For this review, take the finished solid that the model builds, in its own axes (mm). A direction names the side the tool comes from. Coordinates: 2 decimals unless noted, no trailing zeros. Loops run counter-clockwise (first coordinate to the right, second up) from the corner with the lowest first, then second, coordinate; pieces in that order, holes last. Notation, with made-up numbers: M 63,44 L 117,44 A25 ccw 117,69 Z; hole C 33.25,-21.75 d9. An arc over 180 degrees is marked long. Answer as a JSON object with one key per item and string values. Group by question number.
Item 1: Add section D-D (x = 28.5). State the section outline as (y, z) points.
Item 2: Wall thickness on L1, parallel to Z at x = -4, y = 30.5; L2, parallel to Z at x = 0, y = 6.8; L3, parallel to X at y = 8, z = 217: over which ranges is each line inside the solid? List them lowest first. Write a range as from..to.
Item 3: Mouldability with a two-part tool opening along Z and no side actions: class faces 5 (the face through (0, 0, 230)), 6 (the face through (0, 50, 2)), 7 (the face through (0, 30, 5)) as +Z half, -Z half, draft (parallel to the pull), parting line (faces both ways), or undercut.
Item 4: Insertion check: pin 1 (1.5 mm diameter, centred on y = 38.5, z = 26, fed in from +X); pin 2 (2.5 mm diameter, centred on y = 13.5, z = 72, fed in from -X); pin 3 (16.5 mm diameter, centred on x = 2, z = 158, fed in from +Y); pin 4 (5.5 mm diameter, centred on x = -36, z = 31.5, fed in from -Y). Each pin has a flat end and moves straight along its axis. Give the tip position at first contact, or say it passes through.
Item 5: Tool access review of faces 1 (the face through (0, 10, 151)), 2 (the face through (32.5, 16, 2)), 3 (the face through (32.5, 44, 2)), 4 (the face through (32.5, 30, 38)): name each direction out of +Z, -Z, +X, -X, +Y, -Y from which nothing blocks a thin tool from reaching the whole face with its end or side.
Item 6: Add section A-A (y = 0). State the section outline as (x, z) points, then the cut area to 3 significant figures.
Item 7: Add section B-B (z = 50). State the section outline as (x, y) points, then the cut area to 3 significant figures.
Item 8: Add section C-C (y = 34.5). State the section outline as (x, z) points.
from build123d import *

# Parameters (mm, degrees)
SKETCH1_W            = 15
SKETCH1_H            = 20
BOSS_EXTRUDE1_DEPTH  = 230
SKETCH2_W            = 65
SKETCH2_H            = 40
BOSS_EXTRUDE6_DEPTH  = 5
SKETCH7_W            = 75
SKETCH7_H            = 15
BOSS_EXTRUDE7_DEPTH  = 5
SKETCH8_W            = 75
SKETCH8_H            = 15
BOSS_EXTRUDE8_DEPTH  = 5
SKETCH9_W            = 65
SKETCH9_H            = 40
BOSS_EXTRUDE11_DEPTH = 5
CUT_EXTRUDE1_DEPTH   = 240.635139326
SKETCH13_R           = 1.984375
CUT_EXTRUDE2_DEPTH   = 10


with BuildPart() as part:
    # Sketch1 → Boss-Extrude1 (new body)
    with BuildSketch(Plane.XY):
        Rectangle(SKETCH1_W, SKETCH1_H)
    extrude(amount=BOSS_EXTRUDE1_DEPTH)

    # Sketch2 → Boss-Extrude6 (add)
    with BuildSketch(Plane(origin=(0, 0, 0), x_dir=(-1, 0, 0), z_dir=(0, 0, -1))):
        with Locations((0, 30)):
            Rectangle(SKETCH2_W, SKETCH2_H)
    extrude(amount=-BOSS_EXTRUDE6_DEPTH)

    # Sketch7 → Boss-Extrude7 (add)
    with BuildSketch(Plane(origin=(32.5, 0, 0), x_dir=(0, 0, -1), z_dir=(1, 0, 0))):
        with Locations((-37.5, 30)):
            Rectangle(SKETCH7_W, SKETCH7_H)
    extrude(amount=BOSS_EXTRUDE7_DEPTH)

    # Sketch8 → Boss-Extrude8 (add)
    with BuildSketch(Plane.ZY.offset(32.5)):
        with Locations((37.5, 30)):
            Rectangle(SKETCH8_W, SKETCH8_H)
    extrude(amount=BOSS_EXTRUDE8_DEPTH)

    # Sketch9 → Boss-Extrude11 (add)
    with BuildSketch(Plane.XY.offset(75)):
        with Locations((0, 30)):
            Rectangle(SKETCH9_W, SKETCH9_H)
    extrude(amount=-BOSS_EXTRUDE11_DEPTH)

    # Sketch10 → Cut-Extrude1 (cut, through all)
    with BuildSketch(Plane.ZY.offset(7.5)):
        with BuildLine():
            Line((209.843145751, 2), (211.343145751, 2))
            ThreePointArc((211.343145751, 2), (223, 0), (211.343145751, -2))
            Line((211.343145751, -2), (209.843145751, -2))
            Line((209.843145751, -2), (209.843145751, 2))
        make_face()
    extrude(amount=-CUT_EXTRUDE1_DEPTH, mode=Mode.SUBTRACT)

    # Sketch13 → Cut-Extrude2 (cut)
    with BuildSketch(Plane(origin=(0, 10, 0), x_dir=(1, 0, 0), z_dir=(0, 1, 0))):
        with Locations(Location((0, -217, 0), (0, 0, 270))):
            Circle(SKETCH13_R)
    extrude(amount=-CUT_EXTRUDE2_DEPTH, mode=Mode.SUBTRACT)


solid = part.part
From the geometry:
{
 "1": {"outline": "M 10,0 L 50,0 L 50,5 L 10,5 Z; M 10,70 L 50,70 L 50,75 L 10,75 Z"},
 "2": {"L1": "z = 0..5, 70..75", "L2": "z = 0..215.02, 218.98..230", "L3": "x = -7.5..-1.98, 1.98..7.5"},
 "3": {"face 5": "+Z half", "face 6": "draft", "face 7": "undercut"},
 "4": {"pin 1": "passes through", "pin 2": "stops at x = -32.5", "pin 3": "stops at y = 10", "pin 4": "stops at y = 22.5"},
 "5": {"face 1": "+Z, +X, -X, +Y", "face 2": "+Z, -Z, +X, -Y", "face 3": "+Z, -Z, +X, +Y", "face 4": "+Y, -Y"},
 "6": {"outline": "M -7.5,0 L 7.5,0 L 7.5,209.84 L -7.5,209.84 Z; M -7.5,223 L 7.5,223 L 7.5,230 L -7.5,230 Z", "area": "3,250 mm²"},
 "7": {"outline": "M -37.5,22.5 L -32.5,22.5 L -32.5,37.5 L -37.5,37.5 Z; M -7.5,-10 L 7.5,-10 L 7.5,10 L -7.5,10 Z; M 32.5,22.5 L 37.5,22.5 L 37.5,37.5 L 32.5,37.5 Z", "area": "450 mm²"},
 "8": {"outline": "M -37.5,0 L 37.5,0 L 37.5,75 L -37.5,75 Z; hole M -32.5,5 L 32.5,5 L 32.5,70 L -32.5,70 Z"}
}
